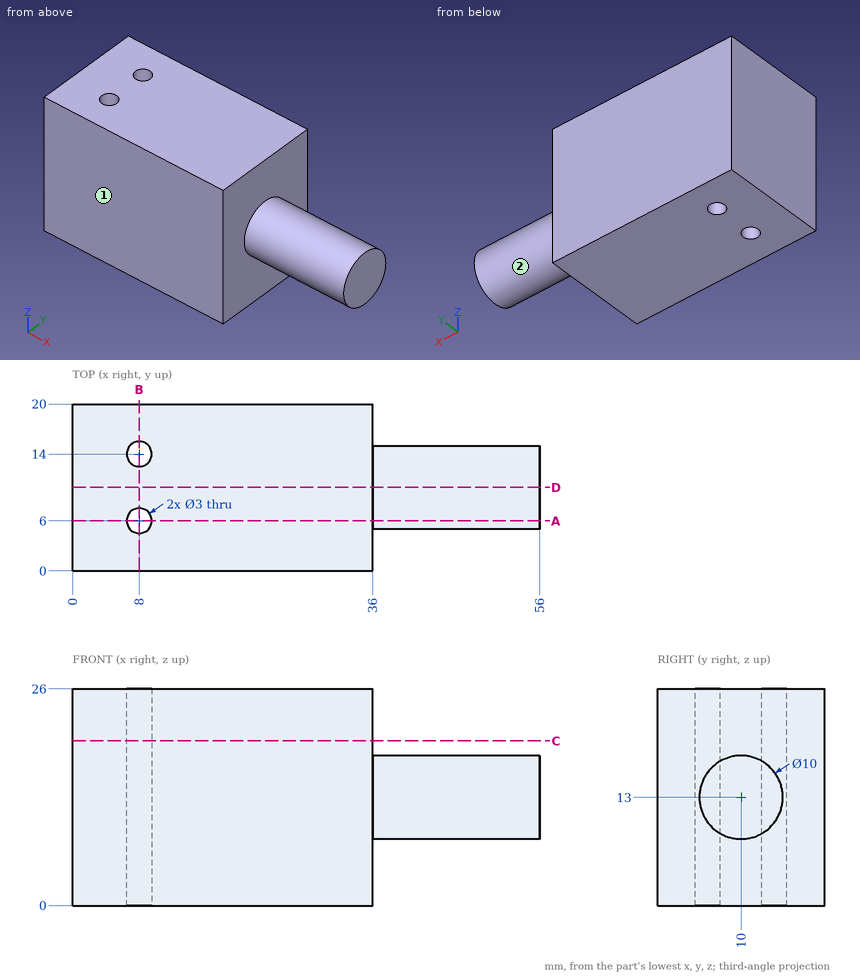
Here's the drawing with two shaded views (mm, measured from the low corner). I have some questions. A direction names the side the tool comes from. Round coordinates to 2 decimals unless told otherwise and drop trailing zeros. Order: outer loops, then holes, each group sorted by start corner. A loop starts at its lowest first (then second) coordinate and runs counter-clockwise, first axis right, second up. Notation, with made-up numbers: M -26,-31.5 L -22,-31.5 A22 ccw -22,-16.5 Z; hole C -26,73.25 d3. An arc over 180 degrees is marked long. Answer in a Markdown table with one row per item.
Item 1: For the marked faces 1 and 2, which set-ups out of +Z, -Z, +X, -X, +Y, -Y let a thin tool reach every point of the face, with its end or its side?
A:
| item | result |
|---|---|
| face 1 | +Z, -Z, +X, -X, -Y |
| face 2 | +X |
Item 2: If I drill on L1, parallel to Y at x = 8, z = 19.25; L2, parallel to X at y = 2.5, z = 6.5; L3, parallel to Z at x = 52, y = 10.5, over which ranges is the centre line in solid material (lowest first)? Write a range as from..to.
A:
| item | result |
|---|---|
| L1 | y = 0..4.5, 7.5..12.5, 15.5..20 |
| L2 | x = 0..36 |
| L3 | z = 8.03..17.97 |
Item 3: Imagine slicing it at C-C, the plane z = 19.75. Write out the boundary of the cut face in (x, y), and give its area (3 significant figures).
A:
| item | result |
|---|---|
| outline | M 0,0 L 36,0 L 36,20 L 0,20 Z; hole C 8,6 d3; hole C 8,14 d3 |
| area | 706 mm2 |
Item 4: I'm going to push flat-ended pins straight in: pin 1 (2.5 mm diameter, centred on x = 8, y = 6, fed in from +Z); pin 2 (2 mm diameter, centred on x = 19.5, y = 8, fed in from -Z); pin 3 (1 mm diameter, centred on x = 49, z = 18, fed in from +Y); pin 4 (10 mm diameter, centred on x = 47, y = 11.5, fed in from -Z). Where does each tip first touch, or does it pass through?
A:
| item | result |
|---|---|
| pin 1 | passes through |
| pin 2 | stops at z = 0 |
| pin 3 | stops at y = 12.18 |
| pin 4 | stops at z = 8 |
Item 5: Imagine slicing it at B-B, the plane x = 8. Write out the boundary of the cut face in (y, z), and give its area (3 significant figures).
A:
| item | result |
|---|---|
| outline | M 0,0 L 4.5,0 L 4.5,26 L 0,26 Z; M 7.5,0 L 12.5,0 L 12.5,26 L 7.5,26 Z; M 15.5,0 L 20,0 L 20,26 L 15.5,26 Z |
| area | 364 mm2 |
Item 6: Imagine slicing it at A-A, the plane y = 6. Write out the boundary of the cut face in (x, z), and give its area (3 significant figures).
A:
| item | result |
|---|---|
| outline | M 0,0 L 6.5,0 L 6.5,26 L 0,26 Z; M 9.5,0 L 36,0 L 36,10 L 56,10 L 56,16 L 36,16 L 36,26 L 9.5,26 Z |
| area | 978 mm2 |
Item 7: Imagine slicing it at D-D, the plane y = 10. Write out the boundary of the cut face in (x, z).
A:
| item | result |
|---|---|
| outline | M 0,0 L 36,0 L 36,8 L 56,8 L 56,18 L 36,18 L 36,26 L 0,26 Z |
